For this review, use the dimensioned drawing (mm, ordinates from the lowest corner) and the shaded views. A direction names the side the tool comes from. Round coordinates to 2 decimals unless told otherwise and drop trailing zeros. Write each loop counter-clockwise with the first axis right and the second up, starting at its lowest first coordinate (ties: lowest second). Pieces come first, ordered by that corner, then holes. Notation, with made-up numbers: M 24.25,34.5 L 55.25,34.5 A19 ccw 55.25,45.5 Z; hole C 55.25,70.25 d2. An arc over 180 degrees is marked long. Use one line per item in the form item = value. Start each with the question number.
Item 1: For the marked faces 1 and 2, list the 3-axis set-ups (+Z, -Z, +X, -X, +Y, -Y) from which the entire face can be reached by the end or side of a thin tool; tool diameter is ignored.
Item 2: Add section B-B (x = 88.9). State the section outline as (y, z) points (1 decimal).
Item 3: For line 1 (X direction, y = 7.75, z = 88.9); line 2 (Y direction, x = 125, z = 166) (1 decimal); line 3 (X direction, y = 5.5, z = 74.5) (1 decimal), list the stretches that pass through material, from the lowest coordinate up. Write a range as [from, to].
Item 4: Add section C-C (y = 13.5). State the section outline as (x, z) points.
Item 5: Draft analysis for pull direction X (two halves, no side actions). For the marked faces 3 and 4, state which applies: released by +X, released by -X, zero draft, split by the parting line, or undercut.
Item 6: Add section A-A (z = 88.9). State the section outline as (x, y) points (1 decimal), and give its area (3 significant figures).
Item 7: For P1, Ø1, axis at y = 7.5, z = 129, coming from the -X side; P2, Ø5, axis at x = 115, y = 13.5, coming from the -Z side; P3, Ø12, axis at y = 12, z = 110, coming from the -X side, all flat-tipped, find the tip position at first contact; note any pin that passes through.
Item 8: Add section D-D (x = 38.5). State the section outline as (y, z) points (1 decimal), and give its area (3 significant figures).
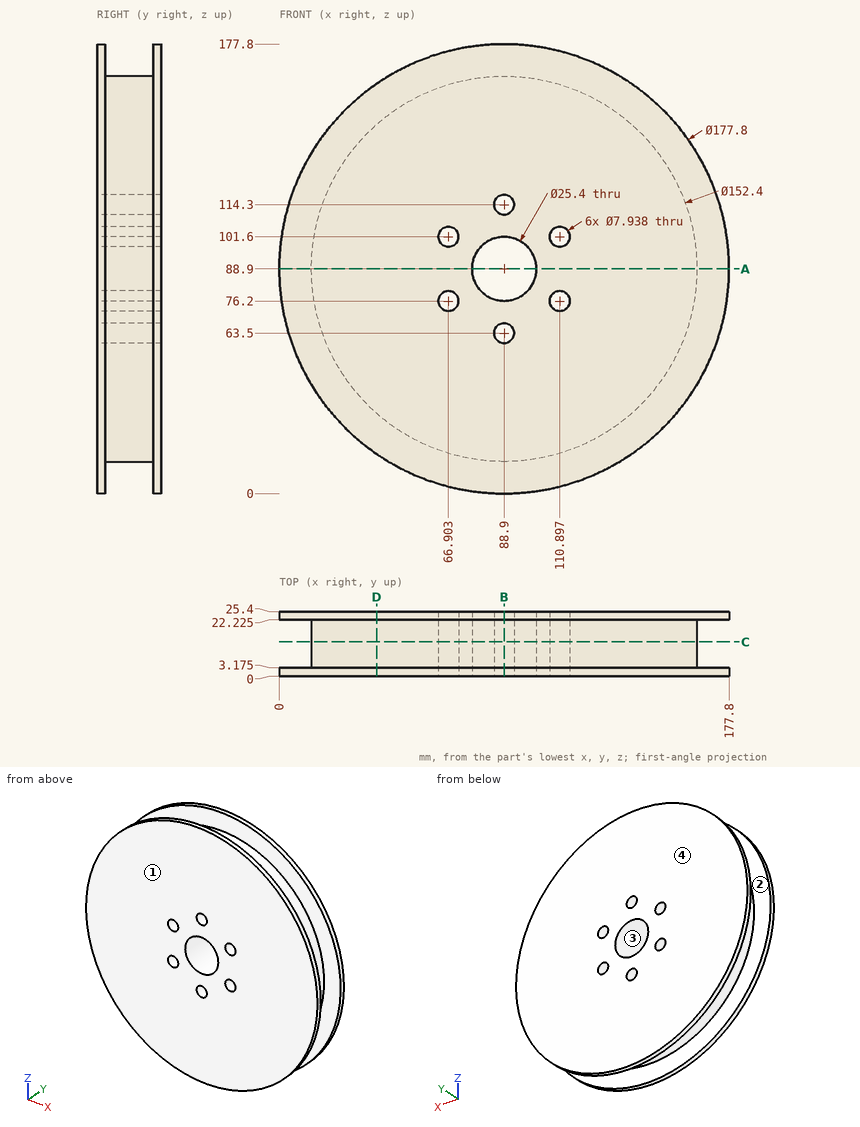
Calculated:
q1.face_1 = +Z, -Z, +X, -X, -Y
q1.face_2 = none
q2.outline = M 0,0 L 3.2,0 L 3.2,12.7 L 22.2,12.7 L 22.2,0 L 25.4,0 L 25.4,59.5 L 0,59.5 Z; M 0,67.5 L 25.4,67.5 L 25.4,76.2 L 0,76.2 Z; M 0,101.6 L 25.4,101.6 L 25.4,110.3 L 0,110.3 Z; M 0,118.3 L 25.4,118.3 L 25.4,177.8 L 22.2,177.8 L 22.2,165.1 L 3.2,165.1 L 3.2,177.8 L 0,177.8 Z
q3.line_1 = [12.7, 76.2], [101.6, 165.1]
q3.line_2 = [0, 3.2], [22.2, 25.4]
q3.line_3 = [14.1, 63.3], [70.5, 107.3], [114.5, 163.7]
q4.outline = C 88.9,88.9 d152.4; hole C 66.9,76.2 d7.94; hole C 66.9,101.6 d7.94; hole C 88.9,88.9 d25.4; hole C 88.9,63.5 d7.94; hole C 88.9,114.3 d7.94; hole C 110.9,76.2 d7.94; hole C 110.9,101.6 d7.94
q5.face_3 = undercut
q5.face_4 = zero draft
q6.outline = M 0,0 L 76.2,0 L 76.2,25.4 L 0,25.4 L 0,22.2 L 12.7,22.2 L 12.7,3.2 L 0,3.2 Z; M 101.6,0 L 177.8,0 L 177.8,3.2 L 165.1,3.2 L 165.1,22.2 L 177.8,22.2 L 177.8,25.4 L 101.6,25.4 Z
q6.area = 3,390 mm^2
q7.P1 = 23.8
q7.P2 = 16.45
q7.P3 = 14.21
q8.outline = M 0,15.7 L 3.2,15.7 L 3.2,31.7 L 22.2,31.7 L 22.2,15.7 L 25.4,15.7 L 25.4,162.1 L 22.2,162.1 L 22.2,146.1 L 3.2,146.1 L 3.2,162.1 L 0,162.1 Z
q8.area = 3,110 mm^2
